Could you check a few things on this drawing? It's one solid part, dimensions in mm from its lowest x, y, z. Coordinates: 2 decimals unless noted, no trailing zeros. Loops run counter-clockwise (first coordinate to the right, second up) from the corner with the lowest first, then second, coordinate; pieces in that order, holes last. Notation, with made-up numbers: (-10.5, 64) -> (30.5, 64) arc R18 cw to (30.5, 75) -> close; hole circle Ø9 at (-15, -38). An arc over 180 degrees is marked (long way). One line per question, with ' | ' between items.
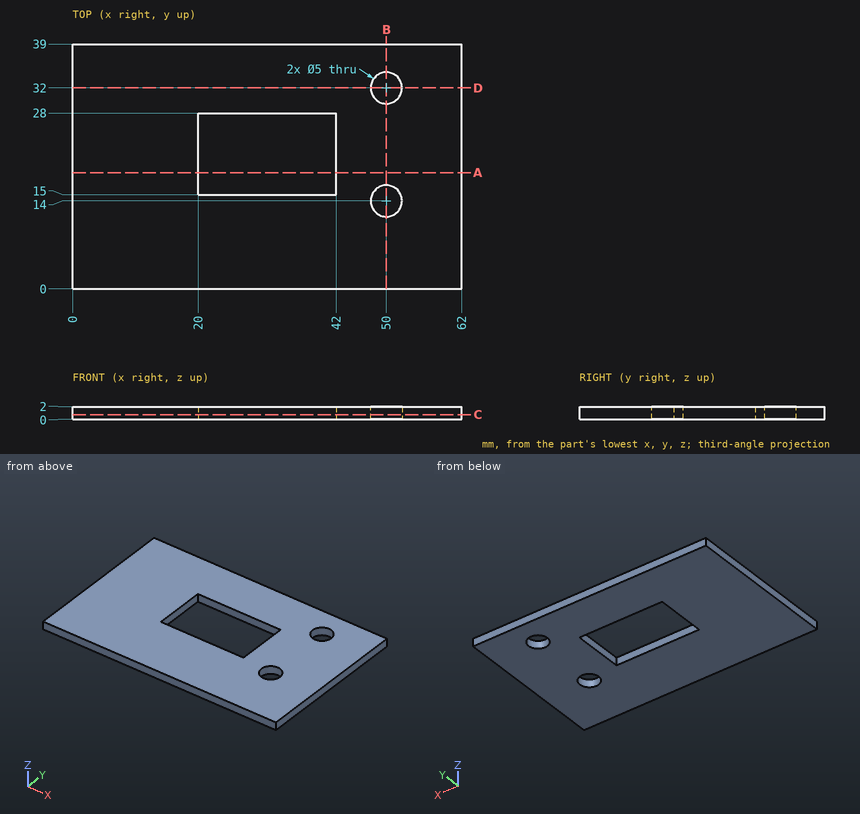
1) If we section it at A-A on y = 18.5: Please give me the cut outline in (x, z).
Data:
outline: (0, 0) -> (20, 0) -> (20, 2) -> (0, 2) -> close; (42, 0) -> (62, 0) -> (62, 2) -> (42, 2) -> close
2) I need wall thicknesses on line 1 along Y through (x, z) = (50, 1.65); line 2 along X through (y, z) = (25, 0.45); line 3 along X through (y, z) = (15.5, 0.2). Which ranges of each line are inside material? Lowest first, please. Write a range as from..to.
Data:
line 1: 0..11.5, 16.5..29.5, 34.5..39 | line 2: 0..20, 42..62 | line 3: 0..20, 42..48, 52..62
3) If we section it at C-C on z = 0.75: Please give me the cut outline in (x, y), and give its area (3 significant figures).
Data:
outline: (0, 0) -> (62, 0) -> (62, 39) -> (0, 39) -> close; hole (20, 15) -> (42, 15) -> (42, 28) -> (20, 28) -> close; hole circle Ø5 at (50, 14); hole circle Ø5 at (50, 32) | area: 2,090 mm²
4) If we section it at B-B on x = 50: Please give me the cut outline in (y, z).
Data:
outline: (0, 0) -> (11.5, 0) -> (11.5, 2) -> (0, 2) -> close; (16.5, 0) -> (29.5, 0) -> (29.5, 2) -> (16.5, 2) -> close; (34.5, 0) -> (39, 0) -> (39, 2) -> (34.5, 2) -> close
5) If we section it at D-D on y = 32: Please give me the cut outline in (x, z), and give its area (3 significant figures).
Data:
outline: (0, 0) -> (47.5, 0) -> (47.5, 2) -> (0, 2) -> close; (52.5, 0) -> (62, 0) -> (62, 2) -> (52.5, 2) -> close | area: 114 mm²
